```python
from build123d import *

# Parameters (mm, degrees)
SKETCH_1_R      = 1.5
EXTRUDE_1_DEPTH = 30
EXTRUDE_2_DEPTH = 2.12


with BuildPart() as part:
    # 草图1 → 凸台-拉伸1 (new body)
    with BuildSketch(Plane(origin=(0, 0, 0), x_dir=(1, 0, 0), z_dir=(0, 1, 0))):
        with Locations(Location((0, 0, 0), (0, 0, 270))):
            Circle(SKETCH_1_R)
    extrude(amount=EXTRUDE_1_DEPTH)

    # 草图3 → 凸台-拉伸2 (add)
    with BuildSketch(Plane.XZ):
        Polygon((3.175426481, 0), (1.58771324, 2.75), (-1.58771324, 2.75), (-3.175426481, 0), (-1.58771324, -2.75), (1.58771324, -2.75), align=None)
    extrude(amount=EXTRUDE_2_DEPTH)


solid = part.part
```
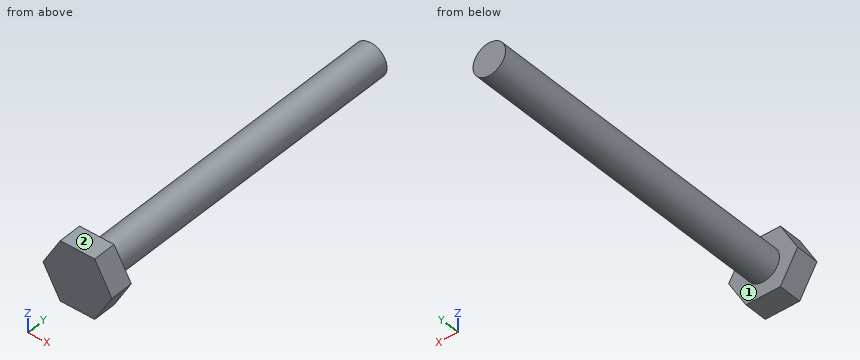
Work out the finished part from the listing and answer in its coordinate system (mm). Face numbers are marked on the shaded views. A direction names the side the tool comes from. Coordinates: 2 decimals unless noted, no trailing zeros. Order: outer loops, then holes, each group sorted by start corner. A loop starts at its lowest first (then second) coordinate and runs counter-clockwise, first axis right, second up. Notation, with made-up numbers: (28, 56.25) - (83, 56.25) arc R20 ccw to (83, 87.25) - close; hole circle Ø5 at (68.5, 3). An arc over 180 degrees is marked (long way). Answer as a JSON object with one key per item and string values.
1. Find section B-B on z = 0.75. Determine the outline of the cut face in (x, y).
Output values:
{"outline": "(-2.74, -2.12) - (2.74, -2.12) - (2.74, 0) - (1.3, 0) - (1.3, 30) - (-1.3, 30) - (-1.3, 0) - (-2.74, 0) - close"}
2. Each of these flat-tipped pins is pushed along its axis until it touches: P1, Ø1, axis at x = 2.5, z = 0, coming from the +Y side; P2, Ø3, axis at y = 18, z = -1, coming from the +X side. Where does it stop, or does it pass through?
Output values:
{"P1": "stops at y = 0", "P2": "stops at x = 1.5"}
3. A tool of negligible diameter and unlimited length cuts with its end or side. For the marked faces 1 and 2, from which of +Z, -Z, +X, -X, +Y, -Y can it reach the whole face along a straight path? Write none if from no direction.
Output values:
{"face 1": "+Y", "face 2": "+Z, +X, -X, +Y, -Y"}
4. Find section A-A on x = 0. Determine the outline of the cut face in (y, z).
Output values:
{"outline": "(-2.12, -2.75) - (0, -2.75) - (0, -1.5) - (30, -1.5) - (30, 1.5) - (0, 1.5) - (0, 2.75) - (-2.12, 2.75) - close"}
5. Consider line 1 (X direction, y = 16.5, z = -0.1); line 2 (Y direction, x = -0.5, z = 2.25); line 3 (X direction, y = 1, z = 0.6). Determine where each line is inside the solid, lowest interval first.
Output values:
{"line 1": "x = -1.5 to 1.5", "line 2": "y = -2.12 to 0", "line 3": "x = -1.37 to 1.37"}
6. Find section D-D on x = -2. Determine the outline of the cut face in (y, z), plus the area to 3 significant figures.
Output values:
{"outline": "(-2.12, -2.04) - (0, -2.04) - (0, 2.04) - (-2.12, 2.04) - close", "area": "8.63 mm²"}
7. Find section C-C on y = 20.5. Determine the outline of the cut face in (x, z).
Output values:
{"outline": "circle Ø3 at (0, 0)"}
